The figure shows three views and two pictorial views of one solid part (mm, origin at its lowest corner). Answer the questions. Coordinates: 2 decimals unless noted, no trailing zeros. Loops run counter-clockwise (first coordinate to the right, second up) from the corner with the lowest first, then second, coordinate; pieces in that order, holes last. Notation, with made-up numbers: (73.5, -36.5) -> (85.5, -36.5) arc R33 cw to (85.5, -4.5) -> close; hole circle Ø5 at (29, 50.25). An arc over 180 degrees is marked (long way). Use a Markdown table: item, result. Add a question column.
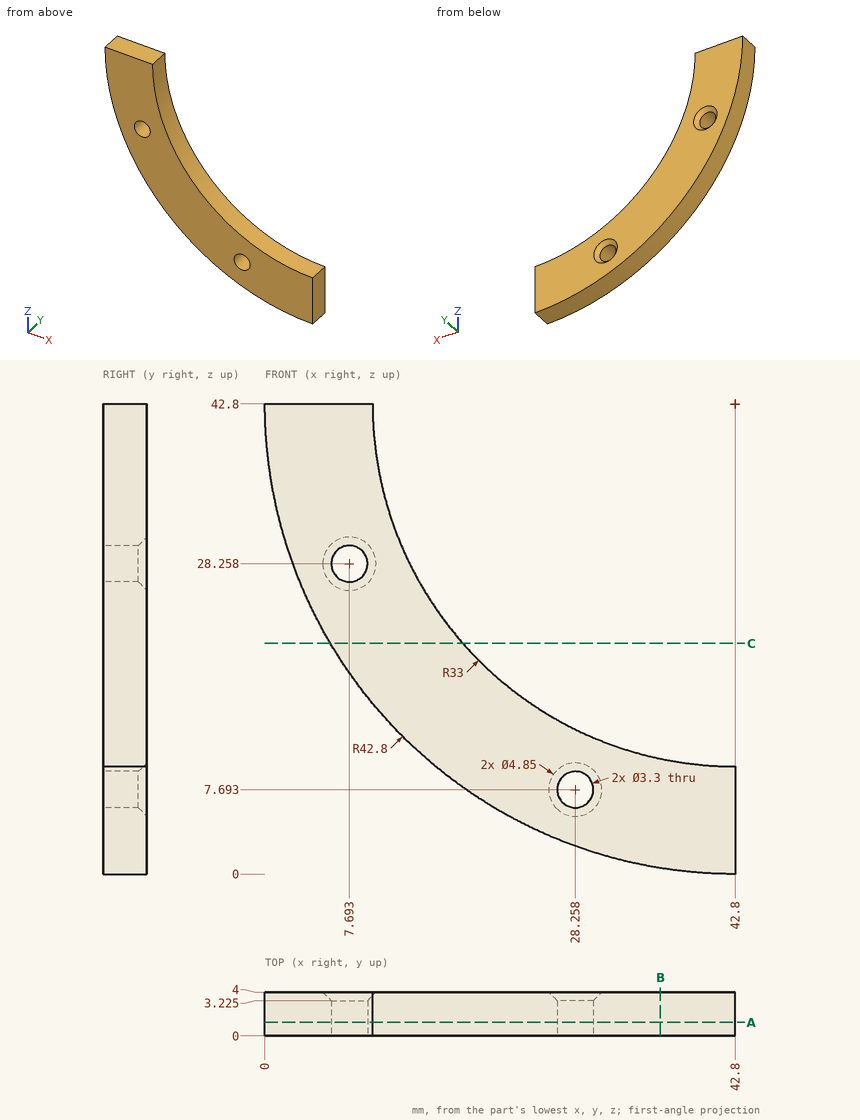
Item 1: Given pin 1 (4.5 mm diameter, centred on x = 28.26, z = 7.69, fed in from +Y); pin 2 (8 mm diameter, centred on x = 30, z = 8, fed in from +Y), each flat-ended and moving along its own axis, determine where each tip first touches the part or whether it passes through.
Item 2: Section A-A (y = 1.25) is taken. Count the separate pieces of the cut face and the enclosed holes in it, then the cut area to 3 significant figures.
Item 3: Section C-C (z = 21) is taken. Determine the outline of the cut face in (x, y) (1 decimal).
Item 4: Find the intervals of material crossed by probe 1 along X at (y, z) = (2.8, 28.5) (1 decimal); probe 2 along X at (y, z) = (1.4, 21) (1 decimal); probe 3 along X at (y, z) = (2, 20) (1 decimal), in increasing order.
Item 5: Section B-B (x = 36) is taken. Determine the outline of the cut face in (y, z).
Output:
| question | item | result |
|---|---|---|
| 1 | pin 1 | stops at y = 3.83 |
| 1 | pin 2 | stops at y = 4 |
| 2 | separate pieces | 1 |
| 2 | enclosed holes | 2 |
| 2 | area | 566 mm2 |
| 3 | outline | (6, 0) -> (18, 0) -> (18, 4) -> (6, 4) -> close |
| 4 | probe 1 | x = 2.5 to 6.1, 9.3 to 13.1 |
| 4 | probe 2 | x = 6 to 18 |
| 4 | probe 3 | x = 6.6 to 18.9 |
| 5 | outline | (0, 0.54) -> (4, 0.54) -> (4, 10.51) -> (0, 10.51) -> close |
